from build123d import *

# Parameters (mm, degrees)
SKETCH1_W           = 100
SKETCH1_H           = 100
BOSS_EXTRUDE1_DEPTH = 30
SKETCH2_W           = 86
SKETCH2_H           = 86
CUT_EXTRUDE1_DEPTH  = 10
SKETCH3_W           = 20
SKETCH3_H           = 15
BOSS_EXTRUDE2_DEPTH = 10


with BuildPart() as part:
    # Sketch1 → Boss-Extrude1 (new body)
    with BuildSketch(Plane(origin=(0, 0, 0), x_dir=(1, 0, 0), z_dir=(0, 1, 0))):
        Rectangle(SKETCH1_W, SKETCH1_H)
    extrude(amount=-BOSS_EXTRUDE1_DEPTH)

    # Sketch2 → Cut-Extrude1 (cut)
    with BuildSketch(Plane(origin=(0, 0, 0), x_dir=(1, 0, 0), z_dir=(0, 1, 0))):
        Rectangle(SKETCH2_W, SKETCH2_H)
    extrude(amount=-CUT_EXTRUDE1_DEPTH, mode=Mode.SUBTRACT)

    # Sketch3 → Boss-Extrude2 (add)
    with BuildSketch(Plane(origin=(50, 0, 0), x_dir=(0, 0, -1), z_dir=(1, 0, 0))):
        with Locations((0, -15)):
            Rectangle(SKETCH3_W, SKETCH3_H)
    extrude(amount=BOSS_EXTRUDE2_DEPTH)


solid = part.part
Geometry check sheet. Reference: the model listing, model coordinates, mm. A direction names the side the tool comes from. Give positions to 0.01 mm unless a question says otherwise; leave off trailing zeros. Write each loop counter-clockwise with the first axis right and the second up, starting at its lowest first coordinate (ties: lowest second). Pieces come first, ordered by that corner, then holes.
1) Cross-section at A-A (y = -2.25). Record the boundary of the cut face in (x, z).
Values follow:
outline: (-50, -50) - (50, -50) - (50, 50) - (-50, 50) - close; hole (-43, -43) - (43, -43) - (43, 43) - (-43, 43) - close
2) Release check for a two-part mould opening along X. For faces 5 (the face through (-50, -15, 1)), 6 (the face through (43, -5, 1)), 7 (the face through (55, -22.5, 0)) record: released by +X, released by -X, zero draft, split by the parting line, or undercut.
Values follow:
face 5: released by -X
face 6: undercut
face 7: zero draft
3) Cross-section at D-D (z = 4). Record the boundary of the cut face in (x, y).
Values follow:
outline: (-50, -30) - (50, -30) - (50, -22.5) - (60, -22.5) - (60, -7.5) - (50, -7.5) - (50, 0) - (43, 0) - (43, -10) - (-43, -10) - (-43, 0) - (-50, 0) - close
4) Set-up check for faces 1 (the face through (55, -7.5, 0)), 2 (the face through (55, -15, 10)), 3 (the face through (-1, -10, -1)), 4 (the face through (55, -15, -10)): record each of +Z, -Z, +X, -X, +Y, -Y from which the full face is reachable in a straight line by a thin tool's end or side.
Values follow:
face 1: +Z, -Z, +X, +Y
face 2: +Z, +X, +Y, -Y
face 3: +Y
face 4: -Z, +X, +Y, -Y
5) Cross-section at C-C (y = -15.75). Record the boundary of the cut face in (x, z), plus the area to 3 significant figures.
Values follow:
outline: (-50, -50) - (50, -50) - (50, -10) - (60, -10) - (60, 10) - (50, 10) - (50, 50) - (-50, 50) - close
area: 10,200 mm2
6) Go/stop test with flat-tipped pins: pin 1 Ø3 at (x, y) = (54, -14.5) entering from -Z; pin 2 Ø12 at (y, z) = (-17, -33) entering from +X; pin 3 Ø5 at (x, z) = (54.5, -2.5) entering from -Y. Record where each tip stops, or that it passes through.
Values follow:
pin 1: stops at z = -10
pin 2: stops at x = 50
pin 3: stops at y = -22.5
7) Cross-section at B-B (z = 22). Record the boundary of the cut face in (x, y), plus the area to 3 significant figures.
Values follow:
outline: (-50, -30) - (50, -30) - (50, 0) - (43, 0) - (43, -10) - (-43, -10) - (-43, 0) - (-50, 0) - close
area: 2,140 mm2
8) Thickness scan on line 1 (Z direction, x = 25, y = -8.25); line 2 (X direction, y = -13.25, z = -19.5). Record the ranges inside material, lowest first.
Values follow:
line 1: z = -50 to -43, 43 to 50
line 2: x = -50 to 50
